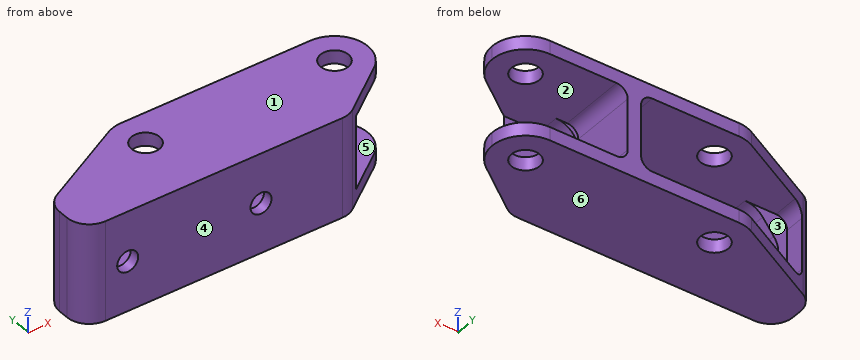
```python
from build123d import *

# Parameters (mm, degrees)
SKETCH1_R           = 3
BOSS_EXTRUDE1_DEPTH = 28.575
CUT_EXTRUDE1_DEPTH  = 19.304
SKETCH9_R           = 3
CUT_EXTRUDE7_DEPTH  = 6.35
SKETCH5_R           = 4
CUT_EXTRUDE3_DEPTH  = 28.575


with BuildPart() as part:
    # Sketch1 → Boss-Extrude1 (new body)
    with BuildSketch(Plane(origin=(0, 0, 0), x_dir=(1, 0, 0), z_dir=(0, 1, 0))):
        Polygon((0, 6.35), (0, 22.225), (0, 28.575), (6.35, 28.575), (88.9, 28.575), (95.25, 28.575), (95.25, 0), (88.9, 0), (6.35, 0), (0, 0), align=None)
        with Locations((12.7, 14.2875)):
            Circle(SKETCH1_R, mode=Mode.SUBTRACT)
        with Locations((50.8, 14.2875)):
            Circle(SKETCH1_R, mode=Mode.SUBTRACT)
    extrude(amount=-BOSS_EXTRUDE1_DEPTH)

    # Sketch2 → Cut-Extrude1 (cut)
    with BuildSketch(Plane(origin=(0, 0, 0), x_dir=(1, 0, 0), z_dir=(0, 1, 0))):
        with BuildLine():
            Line((3.81, 6.985), (3.81, 21.59))
            ThreePointArc((3.81, 21.59), (4.73993597, 23.83506403), (6.985, 24.765))
            Line((6.985, 24.765), (56.515, 24.765))
            ThreePointArc((56.515, 24.765), (58.76006403, 23.83506403), (59.69, 21.59))
            Line((59.69, 21.59), (59.69, 6.985))
            ThreePointArc((59.69, 6.985), (58.76006403, 4.73993597), (56.515, 3.81))
            Line((56.515, 3.81), (6.985, 3.81))
            ThreePointArc((6.985, 3.81), (4.73993597, 4.73993597), (3.81, 6.985))
        make_face()
        with BuildLine():
            Line((63.5, 6.985), (63.5, 21.59))
            ThreePointArc((63.5, 21.59), (64.42993597, 23.83506403), (66.675, 24.765))
            Line((66.675, 24.765), (95.25, 24.765))
            Line((95.25, 24.765), (95.25, 3.81))
            Line((95.25, 3.81), (66.675, 3.81))
            ThreePointArc((66.675, 3.81), (64.42993597, 4.73993597), (63.5, 6.985))
        make_face()
    extrude(amount=-CUT_EXTRUDE1_DEPTH, mode=Mode.SUBTRACT)

    # Sketch9 → Cut-Extrude7 (cut)
    with BuildSketch(Plane(origin=(0, -19.304, 0), x_dir=(1, 0, 0), z_dir=(0, 1, 0))):
        with BuildLine():
            Line((10.793997252, 22.263484848), (7.649092718, 18.135984848))
            ThreePointArc((7.649092718, 18.135984848), (6.35, 14.2875), (7.649092718, 10.439015152))
            Line((7.649092718, 10.439015152), (10.793997252, 6.311515152))
            ThreePointArc((10.793997252, 6.311515152), (13.026694001, 4.469640662), (15.844904534, 3.81))
            Line((15.844904534, 3.81), (47.655095466, 3.81))
            ThreePointArc((47.655095466, 3.81), (50.473305999, 4.469640662), (52.706002748, 6.311515152))
            Line((52.706002748, 6.311515152), (55.850907282, 10.439015152))
            ThreePointArc((55.850907282, 10.439015152), (57.15, 14.2875), (55.850907282, 18.135984848))
            Line((55.850907282, 18.135984848), (52.706002748, 22.263484848))
            ThreePointArc((52.706002748, 22.263484848), (50.473305999, 24.105359338), (47.655095466, 24.765))
            Line((47.655095466, 24.765), (15.844904534, 24.765))
            ThreePointArc((15.844904534, 24.765), (13.026694001, 24.105359338), (10.793997252, 22.263484848))
        make_face()
        with Locations((12.7, 14.2875)):
            Circle(SKETCH9_R, mode=Mode.SUBTRACT)
        with Locations((50.8, 14.2875)):
            Circle(SKETCH9_R, mode=Mode.SUBTRACT)
        with BuildLine():
            ThreePointArc((63.5, 18.415), (65.359871939, 22.905128061), (69.85, 24.765))
            Line((69.85, 24.765), (95.25, 24.765))
            Line((95.25, 24.765), (95.25, 3.81))
            Line((95.25, 3.81), (69.85, 3.81))
            ThreePointArc((69.85, 3.81), (65.359871939, 5.669871939), (63.5, 10.16))
            Line((63.5, 10.16), (63.5, 18.415))
        make_face()
    extrude(amount=-CUT_EXTRUDE7_DEPTH, mode=Mode.SUBTRACT)

    # Sketch5 → Cut-Extrude3 (cut)
    with BuildSketch(Plane(origin=(0, 0, -28.575), x_dir=(-1, 0, 0), z_dir=(0, 0, -1))):
        with BuildLine():
            Line((-95.25, 0), (-95.25, -9.524999828))
            ThreePointArc((-95.25, -9.524999828), (-92.46019203, -2.789807848), (-85.725, 0))
            Line((-85.725, 0), (-95.25, 0))
        make_face()
        with BuildLine():
            Line((-77.893333333, -27.305), (-91.44, -17.145))
            ThreePointArc((-91.44, -17.145), (-94.244419033, -13.78470942), (-95.25, -9.524999828))
            Line((-95.25, -9.524999828), (-95.25, -28.575))
            Line((-95.25, -28.575), (-74.083333333, -28.575))
            ThreePointArc((-74.083333333, -28.575), (-76.091379648, -28.249138943), (-77.893333333, -27.305))
        make_face()
        with BuildLine():
            ThreePointArc((-31.75, 0), (-29.462234044, -0.278825011), (-27.308407483, -1.098975973))
            Line((-27.308407483, -1.098975973), (-3.388938322, -13.707595992))
            ThreePointArc((-3.388938322, -13.707595992), (-0.912848096, -16.044719868), (0, -19.324945344))
            Line((0, -19.324945344), (0, 0))
            Line((0, 0), (-31.75, 0))
        make_face()
        with BuildLine():
            Line((0, -28.575), (0, -22.225))
            ThreePointArc((0, -22.225), (-1.859871939, -26.715128061), (-6.35, -28.575))
            Line((-6.35, -28.575), (0, -28.575))
        make_face()
        with Locations((-31.75, -9.525)):
            Circle(SKETCH5_R)
        with Locations((-85.725, -9.525)):
            Circle(SKETCH5_R)
    extrude(amount=-CUT_EXTRUDE3_DEPTH, mode=Mode.SUBTRACT)


solid = part.part
```
Here's how the part is built. I have some questions about the finished solid (model axes, mm). Face numbers are marked on the shaded views. A direction names the side the tool comes from. Give positions to 0.01 mm unless a question says otherwise; leave off trailing zeros. Order: outer loops, then holes, each group sorted by start corner. A loop starts at its lowest first (then second) coordinate and runs counter-clockwise, first axis right, second up. Notation, with made-up numbers: (-39.75, 20.5) -> (-18.75, 20.5) arc R14 ccw to (-18.75, 28.5) -> close; hole circle Ø1 at (1, 19). An arc over 180 degrees is marked (long way). Use CSV: the item, a comma, the result in double quotes. Start each with the question number.
Item 1: Suppose I cut it at C-C (z = -9). List the corners of the cut face in (x, y) for me (3 decimals), and give its area (3 significant figures).
Item 2: I'm going to push flat-ended pins straight in: P1, Ø7, axis at x = 68, z = -7, coming from the +Y side; P2, Ø12, axis at y = -17.5, z = -14, coming from the +X side; P3, Ø1, axis at x = 73, z = -11.5, coming from the +Y side; P4, Ø5, axis at x = 12.7, z = -14.29, coming from the +Y side. Where does each tip first touch, or does it pass through?
Item 3: Suppose I cut it at D-D (x = 26). List the corners of the cut face in (y, z) for me (3 decimals).
Item 4: If I drill on probe 1 along Z at (x, y) = (70.5, -20) (3 decimals); probe 2 along Z at (x, y) = (12.7, -27.2) (1 decimal); probe 3 along Y at (x, z) = (31.75, -2.35) (3 decimals), over which ranges is the centre line in solid material (lowest first)? Write a range as [from, to].
Item 5: Thinking about a two-plate mould opening in Z: for the marked faces 4, 5 and 6, which applies, pulls with the +Z half, pulls with the -Z half, needs draft (parallel to the pull), parting line crosses it, or undercut?
Item 6: Suppose I cut it at A-A (x = 50.8). List the corners of the cut face in (y, z) for me (1 decimal), and give its area (3 significant figures).
Item 7: On a 3-axis mill with a long thin cutter (end or side, diameter ignored), from which of +Z, -Z, +X, -X, +Y, -Y can I reach the whole of each face in a straight line? I mean the marked faces 1, 2 and 3. Say none if no direction works.
Item 8: Suppose I cut it at B-B (y = -6.75). Give the number of separate pieces and of enclosed holes in the cut face, and give its area (3 significant figures).
Answer block:
1,outline,"(0, -22.225) arc R6.35 ccw to (6.35, -28.575) -> (74.083, -28.575) arc R6.35 ccw to (77.893, -27.305) -> (80.095, -25.654) -> (63.607, -25.654) -> (63.607, -19.304) -> (63.5, -19.304) -> (63.5, 0) -> (59.69, 0) -> (59.69, -19.304) -> (54.754, -19.304) -> (54.754, -25.654) -> (8.746, -25.654) -> (8.746, -19.304) -> (3.81, -19.304) -> (3.81, -13.486) -> (3.389, -13.708) arc R6.35 ccw to (0, -19.325) -> close"
1,area,"420 mm^2"
2,P1,"stops at y = 0"
2,P2,"stops at x = 63.79"
2,P3,"stops at y = -25.65"
2,P4,"passes through"
3,outline,"(-28.575, -28.575) -> (-1.789, -28.575) -> (-1.789, -24.765) -> (-25.654, -24.765) -> (-25.654, -3.81) -> (-1.789, -3.81) -> (-1.789, 0) -> (-28.575, 0) -> close"
4,probe 1,"z = [-28.575, -24.765], [-3.81, 0]"
4,probe 2,"z = [-28.6, -17.3], [-11.3, 0]"
4,probe 3,"y = [-28.575, -13.525], [-5.525, 0]"
5,face 4,"needs draft"
5,face 5,"undercut"
5,face 6,"pulls with the -Z half"
6,outline,"(-28.6, -28.6) -> (0, -28.6) -> (0, -24.8) -> (-19.3, -24.8) -> (-19.3, -23.9) -> (-25.7, -23.9) -> (-25.7, -17.3) -> (-28.6, -17.3) -> close; (-28.6, -11.3) -> (-25.7, -11.3) -> (-25.7, -4.6) -> (-19.3, -4.6) -> (-19.3, -3.8) -> (0, -3.8) -> (0, 0) -> (-28.6, 0) -> close"
6,area,"272 mm^2"
7,face 1,"+Z, +X, -X, +Y, -Y"
7,face 2,"+X, +Y"
7,face 3,"+Y"
8,separate pieces,"5"
8,enclosed holes,"0"
8,area,"597 mm^2"
